Build history of the part. All positions in model axes, mm. A direction names the side the tool comes from. Give positions to 0.01 mm unless a question says otherwise; leave off trailing zeros. Loops run counter-clockwise (first coordinate to the right, second up) from the corner with the lowest first, then second, coordinate; pieces in that order, holes last. Notation, with made-up numbers: (-4, 89) - (32, 89) arc R24 ccw to (32, 121) - close; hole circle Ø3 at (1.5, -18.75). An arc over 180 degrees is marked (long way). Return JSON: item names as keys, results as strings. Group by question number.
1) 3-axis set-ups, long thin cutter, end or side, ignore diameter. For faces 3 (the face through (19, -22, 2)), 4 (the face through (17, -19, 2)): which of +Z, -Z, +X, -X, +Y, -Y reach the whole face in a straight line?
2) Mould opens along X. For faces 1 (the face through (-13.931, -13.865, 4.465)), 2 (the face through (-19, -22, 2)) say: released by +X, released by -X, zero draft, split by the parting line, or undercut.
3) Drop flat-ended pins along their axis: pin 1 (17.5 mm diameter, centred on x = 14, y = 0, fed in from -Z); pin 2 (1 mm diameter, centred on y = 3, z = 2, fed in from +X); pin 3 (4 mm diameter, centred on x = 17, y = 23.5, fed in from -Z); pin 4 (1.9 mm diameter, centred on y = -19, z = 2, fed in from -X). Give the stop position or say it passes through.
4) Drill centre lines: probe 1 along Y at (x, z) = (0, 3.4); probe 2 along X at (y, z) = (-17, 4); probe 3 along X at (y, z) = (-1.5, 1.05). Where is each one in solid material? Low to high. Write a range as from..to.
5) Slice it at B-B (z = 2.3). List the corners of the cut face in (x, y).
6) Slice it at A-A (x = 0). List the corners of the cut face in (y, z), and give its area (3 significant figures).
7) Slice it at C-C (y = -10). Count the separate pieces of the cut face and the enclosed holes in it, and give its area (3 significant figures).
```python
from build123d import *

# Parameters (mm, degrees)
F0_R     = 11
F0_R_2   = 2.6
F1_DEPTH = 4.83
F3_DEPTH = 25
F4_SIZE  = 0.5


with BuildPart() as f1:
    # F0 (on Top) → F1 (new body)
    with BuildSketch(Plane.XY):
        with BuildLine():
            ThreePointArc((20.396078, -22), (27.494384, -12.002451), (30, 0))
            ThreePointArc((30, 0), (-12.002451, 27.494384), (-20.396078, -22))
            Line((-20.396078, -22), (20.396078, -22))
        make_face()
        with Locations((-14, 0)):
            Circle(F0_R, mode=Mode.SUBTRACT)
        with Locations((14, 0)):
            Circle(F0_R, mode=Mode.SUBTRACT)
        with Locations((0, 23)):
            Circle(F0_R_2, mode=Mode.SUBTRACT)
    extrude(amount=F1_DEPTH)

    # F2 (on face) → F3 (cut)
    with BuildSketch(Plane(origin=(0, 0, 0), x_dir=(1, 0, 0), z_dir=(0, 0, -1))):
        with BuildLine():
            ThreePointArc((3, 22), (0, 25), (-3, 22))
            Line((-3, 22), (-3, 17))
            ThreePointArc((-3, 17), (0, 14), (3, 17))
            Line((3, 17), (3, 22))
        make_face()
        with BuildLine():
            ThreePointArc((17, 22), (14, 25), (11, 22))
            Line((11, 22), (11, 17))
            ThreePointArc((11, 17), (14, 14), (17, 17))
            Line((17, 17), (17, 22))
        make_face()
        with BuildLine():
            ThreePointArc((-11, 22), (-14, 25), (-17, 22))
            Line((-17, 22), (-17, 17))
            ThreePointArc((-17, 17), (-14, 14), (-11, 17))
            Line((-11, 17), (-11, 22))
        make_face()
    extrude(amount=-F3_DEPTH, mode=Mode.SUBTRACT)

    # F4
    f4_edges = [f1.edges().sort_by_distance(p)[0] for p in [
        (0, 30, 0),
        (18.698039, -22, 0),
        (17, -19.5, 0),
        (14, -14, 0),
        (11, -19.5, 0),
        (7, -22, 0),
        (3, -19.5, 0),
        (0, -14, 0),
        (-3, -19.5, 0),
        (-7, -22, 0),
        (-11, -19.5, 0),
        (-14, -14, 0),
        (-17, -19.5, 0),
        (-18.698039, -22, 0),
        (-25, 0, 0),
        (3, 0, 0),
        (-2.6, 23, 0),
        (0, 30, 4.83),
        (18.698039, -22, 4.83),
        (17, -19.5, 4.83),
        (14, -14, 4.83),
        (11, -19.5, 4.83),
        (7, -22, 4.83),
        (3, -19.5, 4.83),
        (0, -14, 4.83),
        (-3, -19.5, 4.83),
        (-7, -22, 4.83),
        (-11, -19.5, 4.83),
        (-14, -14, 4.83),
        (-17, -19.5, 4.83),
        (-18.698039, -22, 4.83),
        (-25, 0, 4.83),
        (3, 0, 4.83),
        (-2.6, 23, 4.83),
    ]]
    chamfer(f4_edges, length=F4_SIZE)


solid = f1.part
```
Results:
{
 "1": {"face 3": "+Z, -Z, +X, -X, -Y", "face 4": "+Z, -Z, -Y"},
 "2": {"face 1": "undercut", "face 2": "zero draft"},
 "3": {"pin 1": "through", "pin 2": "x = 29.9", "pin 3": "z = 0", "pin 4": "x = -23.96"},
 "4": {"probe 1": "-14..20.4, 25.6..30", "probe 2": "-24.72..-17, -11..-3, 3..11, 17..24.72", "probe 3": "-29.96..-24.9, -3.1..3.1, 24.9..29.96"},
 "5": {"outline": "(-20.4, -22) - (-17, -22) - (-17, -17) arc R3 cw to (-11, -17) - (-11, -22) - (-3, -22) - (-3, -17) arc R3 cw to (3, -17) - (3, -22) - (11, -22) - (11, -17) arc R3 cw to (17, -17) - (17, -22) - (20.4, -22) arc R30 ccw to (30, 0) arc R30 ccw (long way) to start; hole circle Ø22 at (-14, 0); hole circle Ø5.2 at (0, 23); hole circle Ø22 at (14, 0)"},
 "6": {"outline": "(-14, 0.5) - (-13.5, 0) - (19.9, 0) - (20.4, 0.5) - (20.4, 4.33) - (19.9, 4.83) - (-13.5, 4.83) - (-14, 4.33) - close; (25.6, 0.5) - (26.1, 0) - (29.5, 0) - (30, 0.5) - (30, 4.33) - (29.5, 4.83) - (26.1, 4.83) - (25.6, 4.33) - close", "area": "186 mm2"},
 "7": {"separate pieces": "3", "enclosed holes": "0", "area": "182 mm2"}
}
